Check sheet for the modelled part. Datum: model origin and axes. Units: mm. Face numbers are marked on the shaded views. Coordinates: 2 decimals unless noted, no trailing zeros. Write each loop counter-clockwise with the first axis right and the second up, starting at its lowest first coordinate (ties: lowest second). Pieces come first, ordered by that corner, then holes. Notation, with made-up numbers: (8, -16) - (55, -16) arc R19 ccw to (55, 21) - close; hole circle Ø8 at (-26, -39). An arc over 180 degrees is marked (long way). Use one line per item in the form item = value. Start each with the question number.
1. Cross-section at A-A on z = 0. Record the boundary of the cut face in (x, y).
2. Draft check along Z on the marked faces 1, 2 and 3. Enter one of: +Z half, -Z half, draft (parallel to the pull), parting line (faces both ways), or undercut.
3. Cross-section at C-C on y = 0.45. Record the boundary of the cut face in (x, z), then the cut area to 3 significant figures.
4. Scan lines: line 1 along Z through (x, y) = (0, 1.3); line 2 along Z through (x, y) = (0.5, 0.95); line 3 along Z through (x, y) = (3.5, 1.55). Record each from-to range of solid material in increasing order.
5. Go/stop test with flat-tipped pins: pin 1 Ø1 at (x, y) = (-3, 0.5) entering from -Z; pin 2 Ø2.5 at (x, z) = (0, 0) entering from +Y. Record where each tip stops, or that it passes through.
6. Cross-section at B-B on x = 0. Record the boundary of the cut face in (y, z), then the cut area to 3 significant figures.
```python
from build123d import *

# Parameters (mm, degrees)
F0_R     = 4.5
F1_DEPTH = 2
F2_R     = 2
F3_DEPTH = 2.001
F4_SIZE  = 0.1


with BuildPart() as f1:
    # F0 (on Front) → F1 (new body)
    with BuildSketch(Plane.XZ):
        Circle(F0_R)
    extrude(amount=-F1_DEPTH)

    # F2 (on face) → F3 (cut, through all)
    with BuildSketch(Plane.XZ):
        Circle(F2_R)
    extrude(amount=-F3_DEPTH, mode=Mode.SUBTRACT)

    # F4
    f4_edges = [f1.edges().sort_by_distance(p)[0] for p in [
        (-2, 0, 0),
        (-4.5, 0, 0),
        (-2, 2, 0),
    ]]
    chamfer(f4_edges, length=F4_SIZE)


solid = f1.part
```
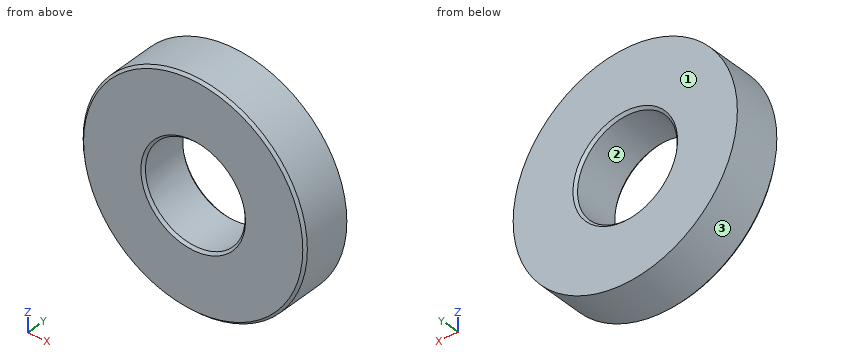
Final values:
q1.outline = (-4.5, 0.1) - (-4.4, 0) - (-2.1, 0) - (-2, 0.1) - (-2, 1.9) - (-2.1, 2) - (-4.5, 2) - close; (2, 0.1) - (2.1, 0) - (4.4, 0) - (4.5, 0.1) - (4.5, 2) - (2.1, 2) - (2, 1.9) - close
q2.face_1 = draft
q2.face_2 = undercut
q2.face_3 = parting line
q3.outline = circle Ø9 at (0, 0); hole circle Ø4 at (0, 0)
q3.area = 51.1 mm²
q4.line_1 = -4.5 to -2, 2 to 4.5
q4.line_2 = -4.47 to -1.94, 1.94 to 4.47
q4.line_3 = -2.83 to 2.83
q5.pin_1 = -3.74
q5.pin_2 = through
q6.outline = (0, -4.4) - (0.1, -4.5) - (2, -4.5) - (2, -2.1) - (1.9, -2) - (0.1, -2) - (0, -2.1) - close; (0, 2.1) - (0.1, 2) - (1.9, 2) - (2, 2.1) - (2, 4.5) - (0.1, 4.5) - (0, 4.4) - close
q6.area = 9.97 mm²
